Autodesk Inventor part; units mm, degrees
ref_plane "YZ Plane" through (0, 0, 0) normal (1, 0, 0) x (0, 1, 0)
ref_plane "XZ Plane" through (0, 0, 0) normal (0, 1, 0) x (-1, 0, 0)
ref_plane "XY Plane" through (0, 0, 0) normal (0, 0, 1) x (1, 0, 0)
sketch "Sketch2" plane through (0, 0, 0) normal (0, 0, 1) x (1, 0, 0)
  line L0 (-75, -25) -> (75, -25)
  line L1 (75, -25) -> (75, 25)
  line L2 (75, 25) -> (-75, 25)
  line L3 (-75, 25) -> (-75, -25)
  line L4 (-75, -25) -> (75, 25) construction
  line L5 (75, -25) -> (-75, 25) construction
  point P0 (0, 0)
  dimension "d1" = 150
  dimension "d2" = 50
extrude "Extrusion1" add sketch "Sketch2" along normal mid plane 10
sketch "Sketch3" plane through (0, 0, 5) normal (0, 0, 1) x (1, 0, 0)
  line L0 (-75, 25) -> (-75, -25)
  line L1 (75, 25) -> (-75, 25)
  point P0 (0, 0)
  point P1 (-65, 0)
  dimension "d40" = 10
  dimension "d43" = 25
hole "Hole1" at (-65, 0, 5) direction (0, 0, -1) diameter 5.5 depth 14.2 tip angle 118 countersink diameter 10.4 countersink angle 90
sketch "Sketch4" plane through (0, 0, 5) normal (0, 0, 1) x (1, 0, 0)
  line L0 (-75, 25) -> (-75, -25)
  line L1 (75, 25) -> (-75, 25)
  point P0 (0, 0)
  point P1 (-45, 5)
  dimension "d41" = 30
  dimension "d42" = 20
hole "Hole2" at (-45, 5, 5) direction (0, 0, -1) diameter 6.6 depth 14.2 tip angle 118 countersink diameter 12.6 countersink angle 90
sketch "Sketch5" plane through (0, 0, 5) normal (0, 0, 1) x (1, 0, 0)
  line L0 (-75, 25) -> (-75, -25)
  line L1 (75, 25) -> (-75, 25)
  point P0 (0, 0)
  point P1 (-25, 5)
  dimension "d44" = 50
  dimension "d45" = 20
hole "Hole3" at (-25, 5, 5) direction (0, 0, -1) diameter 9 depth 14.2 tip angle 118 countersink diameter 17.3 countersink angle 90
properties part number "홀간 거리 확인 파트-10" material "SS400"
Geometry: final body of the model. Coordinates: model frame, mm. Round coordinates to 2 decimals unless told otherwise and drop trailing zeros. Loops run counter-clockwise (first coordinate to the right, second up) from the corner with the lowest first, then second, coordinate; pieces in that order, holes last. Notation, with made-up numbers: (8.5, -18.75) -> (67.5, -18.75) arc R14 ccw to (67.5, 1.25) -> close; hole circle Ø1 at (45.25, 15.25). An arc over 180 degrees is marked (long way). Write each question's results on one line, items separated by ' | '.
Item 1: Pull-direction query (Y, two-part tool) for faces 1 (the face through (-67.727, 0.358, -1.278)), 2 (the face through (-1, 0, 5)), 3 (the face through (1, 25, 0)); classes: pulls with the +Y half, pulls with the -Y half, needs draft (parallel to the pull), parting line crosses it, or undercut.
Answers below:
face 1: undercut | face 2: needs draft | face 3: pulls with the +Y half
Item 2: Cut plane A-A on x = -25. Return the cut outline in (y, z), and give its area (3 significant figures).
Answers below:
outline: (-25, -5) -> (0.5, -5) -> (0.5, 0.85) -> (-3.65, 5) -> (-25, 5) -> close; (9.5, -5) -> (25, -5) -> (25, 5) -> (13.65, 5) -> (9.5, 0.85) -> close | area: 393 mm²
Item 3: Line query: probe 1 along X at (y, z) = (5, -0.25); probe 2 along X at (y, z) = (0, -0.5); probe 3 along Y at (x, z) = (-25, -1). Output: solid intervals per line, ascending. Write a range as [from, to].
Answers below:
probe 1: x = [-75, -48.3], [-41.7, -29.5], [-20.5, 75] | probe 2: x = [-75, -67.75], [-62.25, 75] | probe 3: y = [-25, 0.5], [9.5, 25]
Item 4: Cut plane C-C on x = -65. Return the cut outline in (y, z), and give its area (3 significant figures).
Answers below:
outline: (-25, -5) -> (-2.75, -5) -> (-2.75, 2.55) -> (-5.2, 5) -> (-25, 5) -> close; (2.75, -5) -> (25, -5) -> (25, 5) -> (5.2, 5) -> (2.75, 2.55) -> close | area: 439 mm²
Item 5: Pin query (flat end, axial travel): pin 1 Ø14.5 at (x, y) = (-25, 5) entering from +Z; pin 2 Ø3.5 at (x, y) = (-65, 0) entering from +Z. Return the tip coordinate at first contact, or that it passes through.
Answers below:
pin 1: stops at z = 3.6 | pin 2: passes through
Item 6: Cut plane B-B on z = -3.5. Return the cut outline in (x, y), and give its area (3 significant figures).
Answers below:
outline: (-75, -25) -> (75, -25) -> (75, 25) -> (-75, 25) -> close; hole circle Ø5.5 at (-65, 0); hole circle Ø6.6 at (-45, 5); hole circle Ø9 at (-25, 5) | area: 7,380 mm²
